Design review of the part built by this model. Coordinates are the model's own, in mm. A direction names the side the tool comes from. Coordinates: 2 decimals unless noted, no trailing zeros. Order: outer loops, then holes, each group sorted by start corner. A loop starts at its lowest first (then second) coordinate and runs counter-clockwise, first axis right, second up. Notation, with made-up numbers: M 51.25,41.5 L 62.25,41.5 A34 cw 62.25,74.5 Z; hole C -8,81 d9. An arc over 180 degrees is marked long. Answer as a JSON object with one key per item and string values.
from build123d import *

# Parameters (mm, degrees)
F0_W     = 98
F0_H     = 65
F1_DEPTH = 44
F2_W     = 14
F2_H     = 12
F3_DEPTH = 25
F5_DEPTH = 44.001


with BuildPart() as f1:
    # F0 (on Front) → F1 (new body)
    with BuildSketch(Plane.XZ):
        Rectangle(F0_W, F0_H)
    extrude(amount=F1_DEPTH)

    # F2 (on face) → F3 (cut)
    with BuildSketch(Plane.XZ.offset(44)):
        with Locations((-42, 26.5)):
            Rectangle(F2_W, F2_H)
        with Locations((42, 26.5)):
            Rectangle(F2_W, F2_H)
    extrude(amount=-F3_DEPTH, mode=Mode.SUBTRACT)

    # F4 (on face) → F5 (cut, through all)
    with BuildSketch(Plane.XZ.offset(44)):
        Polygon((49, 7.5), (15, -32.5), (49, -32.5), align=None)
        Polygon((-15, -32.5), (-49, 7.5), (-49, -32.5), align=None)
    extrude(amount=-F5_DEPTH, mode=Mode.SUBTRACT)


solid = f1.part
1) Mouldability with a two-part tool opening along Z and no side actions: class faces 1 (the flat face through (-42, -19, 27)), 2 (the flat face through (-31.76, -22.31, -12.78)), 3 (the flat face through (-1, -22, 32.5)) as released by +Z, released by -Z, zero draft, split by the parting line, or undercut.
Taken from the geometry:
{"face 1": "zero draft", "face 2": "released by -Z", "face 3": "released by +Z"}
2) Add section B-B (y = -28.5). State the section outline as (x, z) points.
Taken from the geometry:
{"outline": "M -49,7.5 L -15,-32.5 L 15,-32.5 L 49,7.5 L 49,20.5 L 35,20.5 L 35,32.5 L -35,32.5 L -35,20.5 L -49,20.5 Z"}
3) Add section C-C (z = 2.5). State the section outline as (x, y) points, and give its area (3 significant figures).
Taken from the geometry:
{"outline": "M -44.75,-44 L 44.75,-44 L 44.75,0 L -44.75,0 Z", "area": "3,940 mm2"}
4) Add section A-A (x = 40.5). State the section outline as (y, z) points.
Taken from the geometry:
{"outline": "M -44,-2.5 L 0,-2.5 L 0,32.5 L -19,32.5 L -19,20.5 L -44,20.5 Z"}
5) Add section D-D (y = -16). State the section outline as (x, z) points, and give its area (3 significant figures).
Taken from the geometry:
{"outline": "M -49,7.5 L -15,-32.5 L 15,-32.5 L 49,7.5 L 49,32.5 L -49,32.5 Z", "area": "5,010 mm2"}
6) Insertion check: pin 1 Ø11 at (x, y) = (-45, -31.5) entering from +Z; pin 2 Ø12 at (x, y) = (-25, -15) entering from -Z; pin 3 Ø2 at (x, y) = (-35.5, -14) entering from -Z. Each pin has a flat end and moves straight along its axis. Give the tip position at first contact, or say it passes through.
Taken from the geometry:
{"pin 1": "stops at z = 20.5", "pin 2": "stops at z = -27.79", "pin 3": "stops at z = -9.56"}
7) To check wall thickness, follow L1, parallel to X at y = -6.5, z = 4.5; L2, parallel to X at y = -3.5, z = 2.5; L3, parallel to Z at x = 33, y = -33. State the ranges of each line that lie inside material, in increasing order.
Taken from the geometry:
{"L1": "x = -46.45 to 46.45", "L2": "x = -44.75 to 44.75", "L3": "z = -11.32 to 32.5"}
8) Tool access review of faces 4 (the flat face through (-42, -32, 20.5)), 5 (the flat face through (35, -32, 26)), 6 (the flat face through (49, -17, 17)): name each direction out of +Z, -Z, +X, -X, +Y, -Y from which nothing blocks a thin tool from reaching the whole face with its end or side.
Taken from the geometry:
{"face 4": "+Z, -X, -Y", "face 5": "+Z, +X, -Y", "face 6": "+Z, -Z, +X, +Y, -Y"}
